```python
from build123d import *

# Parameters (mm, degrees)
SKETCH1_W                      = 78
SKETCH1_H                      = 70
BOSS_EXTRUDE1_DEPTH            = 12
F_17_0_17_DIAMETER_HOLE1_D     = 17
F_17_0_17_DIAMETER_HOLE1_DEPTH = 25
F_17_0_17_DIAMETER_HOLE1_TIP   = 5.107315262
F_3_0_3_DIAMETER_HOLE1_D       = 3
CUT_EXTRUDE1_REACH             = 83.025
SKETCH8_R                      = 14
CUT_EXTRUDE2_DEPTH             = 58.636793906


with BuildPart() as part:
    # Sketch1 → Boss-Extrude1 (new, symmetric)
    with BuildSketch(Plane.XY):
        Rectangle(SKETCH1_W, SKETCH1_H)
    extrude(amount=BOSS_EXTRUDE1_DEPTH, both=True)

    # Ø17.0 (17) Diameter Hole1
    with Locations(Plane(origin=(0, 35, 0), x_dir=(1, 0, 0), z_dir=(0, 1, 0))):
        with Locations((0, 0)):
            Hole(F_17_0_17_DIAMETER_HOLE1_D / 2, depth=F_17_0_17_DIAMETER_HOLE1_DEPTH)
            with Locations((0, 0, -(F_17_0_17_DIAMETER_HOLE1_DEPTH + F_17_0_17_DIAMETER_HOLE1_TIP / 2))):  # 118° drill point
                Cone(0, F_17_0_17_DIAMETER_HOLE1_D / 2, F_17_0_17_DIAMETER_HOLE1_TIP, mode=Mode.SUBTRACT)

    # Ø3.0 (3) Diameter Hole1 (through all)
    with Locations(Plane.XY.offset(12)):
        with Locations((8.5, 23)):
            Hole(F_3_0_3_DIAMETER_HOLE1_D / 2)

    # Sketch8 → Cut-Extrude1 (cut, up to next)
    with BuildSketch(Plane(origin=(0, 35, 0), x_dir=(1, 0, 0), z_dir=(0, 1, 0)), mode=Mode.PRIVATE) as cut_extrude1_sk1:
        with Locations((-47.8, 0)):
            Circle(SKETCH8_R)
    cut_extrude1_tool1 = extrude(cut_extrude1_sk1.sketch, amount=-CUT_EXTRUDE1_REACH, mode=Mode.PRIVATE) & part.part
    # Sketch8 → Cut-Extrude1 (cut, up to next)
    with BuildSketch(Plane(origin=(0, 35, 0), x_dir=(1, 0, 0), z_dir=(0, 1, 0)), mode=Mode.PRIVATE) as cut_extrude1_sk2:
        with Locations((47.8, 0)):
            Circle(SKETCH8_R)
    cut_extrude1_tool2 = extrude(cut_extrude1_sk2.sketch, amount=-CUT_EXTRUDE1_REACH, mode=Mode.PRIVATE) & part.part
    add(cut_extrude1_tool1.solids().sort_by_distance((-47.8, 35, 0))[0], mode=Mode.SUBTRACT)
    add(cut_extrude1_tool2.solids().sort_by_distance((47.8, 35, 0))[0], mode=Mode.SUBTRACT)

    # Sketch9 → Cut-Extrude2 (cut, through all)
    with BuildSketch(Plane.XY.offset(12)):
        Polygon((-27, -35), (27, -35), (27, -32), (24, -32), (24, -29), (21, -29), (21, -26), (18, -26), (18, -23), (15, -23), (15, -20), (12, -20), (12, -17), (9, -17), (9, -14), (6, -14), (6, -11), (3, -11), (3, -8), (0, -8), (-3, -8), (-3, -11), (-6, -11), (-6, -14), (-9, -14), (-9, -17), (-12, -17), (-12, -20), (-15, -20), (-15, -23), (-18, -23), (-18, -26), (-21, -26), (-21, -29), (-24, -29), (-24, -32), (-27, -32), align=None)
    extrude(amount=-CUT_EXTRUDE2_DEPTH, mode=Mode.SUBTRACT)


solid = part.part
```
Could you check a few things on this model? Use its own coordinates, in mm. A direction names the side the tool comes from. Coordinates: 2 decimals unless noted, no trailing zeros. Loops run counter-clockwise (first coordinate to the right, second up) from the corner with the lowest first, then second, coordinate; pieces in that order, holes last. Notation, with made-up numbers: M 47.25,71.25 L 58.25,71.25 A32 ccw 58.25,102.25 Z; hole C 88.25,-7.75 d7. An arc over 180 degrees is marked long. Put each result on its own line as item: value. Start each with the question number.
(1) Suppose I cut it at B-B on x = 14. Please give me the cut outline in (y, z).
(2) Suppose I cut it at D-D on y = 23. Please give me the cut outline in (x, z).
(3) Will these pins go through, and if not, where does the flat tip stop? P1, Ø2.5, axis at x = -22, z = -2.5, coming from the -Y side; P2, Ø2.5, axis at y = -21.5, z = 4.5, coming from the -X side; P3, Ø2.5, axis at y = -21.5, z = -1, coming from the +X side.
(4) I need wall thicknesses on line 1 (Z direction, x = 0, y = 16); line 2 (Y direction, x = 8.5, z = -2.75); line 3 (Y direction, x = 13.5, z = -7.75). Which ranges of each line are inside material? Lowest first, please. Write a range as from..to.
(5) Thinking about a two-plate mould opening in X: for faces 3 (the face through (-33.8, 0.5, 0.2)), 4 (the face through (-1, 0, 12)), 5 (the face through (3, -10, 0)), which applies, pulls with the +X half, pulls with the -X half, needs draft (parallel to the pull), parting line crosses it, or undercut?
(6) Suppose I cut it at C-C on y = 7.5. Please give me the cut outline in (x, z).
(7) Suppose I cut it at A-A on y = -9. Please give me the cut outline in (x, z), then the cut area to 3 significant figures.
(8) For faces 1 (the face through (-1, 0, -12)), 2 (the face through (9, -16, 0)), which set-ups out of +Z, -Z, +X, -X, +Y, -Y let a thin tool reach every point of the face, with its end or its side?
Solutions:
1. outline: M -20,-12 L 35,-12 L 35,12 L -20,12 Z
2. outline: M -39,-12 L 7,-12 L 7,-4.82 A8.5 cw long 7,4.82 L 7,12 L -39,12 L -39,10.89 A14 cw -39,-10.89 Z; M 10,-12 L 39,-12 L 39,-10.89 A14 cw 39,10.89 L 39,12 L 10,12 Z
3. P1: stops at y = -29
3. P2: stops at x = -35.04
3. P3: stops at x = 33.98
4. line 1: z = -12..-8.5, 8.5..12
4. line 2: y = -14..21.5, 24.5..35
4. line 3: y = -20..35
5. face 3: pulls with the -X half
5. face 4: needs draft
5. face 5: undercut
6. outline: M -39,-12 L 39,-12 L 39,-10.89 A14 cw 39,10.89 L 39,12 L -39,12 L -39,10.89 A14 cw -39,-10.89 Z; hole C 0,0 d8.68
7. outline: M -39,-12 L -3,-12 L -3,12 L -39,12 L -39,10.89 A14 cw -39,-10.89 Z; M 3,-12 L 39,-12 L 39,-10.89 A14 cw 39,10.89 L 39,12 L 3,12 Z
7. area: 1,570 mm2
8. face 1: -Z, +X, -X, +Y, -Y
8. face 2: +Z, -Z, -Y
